Work out the finished part from the listing and answer in its coordinate system (mm). Face numbers are marked on the shaded views. Round coordinates to 2 decimals unless told otherwise and drop trailing zeros. Write each loop counter-clockwise with the first axis right and the second up, starting at its lowest first coordinate (ties: lowest second). Pieces come first, ordered by that corner, then holes.
1. Determine the mould class of the marked faces 1, 2 and 3 for opening direction X: pulls with the +X half, pulls with the -X half, needs draft (parallel to the pull), parting line crosses it, or undercut.
2. Straight lines are drawn through the part: probe 1 along Z at (x, y) = (57, -16); probe 2 along X at (y, z) = (-21, 25); probe 3 along X at (y, z) = (-22, 24). For each, find the intervals that lie inside material, in ascending order.
3. Find section C-C (y = -4). Write down the section's boundary in (x, z).
4. Find section A-A (x = 28). Write down the section's boundary in (y, z).
5. Flat-ended cylindrical pins translate along their axes: pin 1 Ø4 at (y, z) = (-20, 31.5) entering from -X; pin 2 Ø1 at (y, z) = (-24, 36.5) entering from -X; pin 3 Ø1.5 at (x, z) = (30, 15) entering from +Y. Find the tip coordinate at first contact, or state that the pin passes through.
6. Find section B-B (z = 8). Write down the section's boundary in (x, y), and give its area (3 significant figures).
7. Find section D-D (x = 54). Write down the section's boundary in (y, z), and give its area (3 significant figures).
```python
from build123d import *

# Parameters (mm, degrees)
F0_W     = 59.392195
F0_H     = 41.705828
F1_DEPTH = 3.048
F2_R     = 7.737953
F3_DEPTH = 41.656
F4_R     = 5.430673
F5_DEPTH = 50.8


with BuildPart() as f1:
    # F0 (on Top) → F1 (new body)
    with BuildSketch(Plane.XY):
        with Locations((29.696097, -20.852914)):
            Rectangle(F0_W, F0_H)
    extrude(amount=F1_DEPTH)

    # F2 (on face) → F3 (join)
    with BuildSketch(Plane.XY.offset(3.048)):
        with Locations((23.27165, -19.919522)):
            Circle(F2_R)
    extrude(amount=F3_DEPTH)

    # F4 (on face) → F5 (cut)
    with BuildSketch(Plane.XY.offset(44.704)):
        with Locations((23.27165, -19.919522)):
            Circle(F4_R)
    extrude(amount=-F5_DEPTH, mode=Mode.SUBTRACT)


solid = f1.part
```
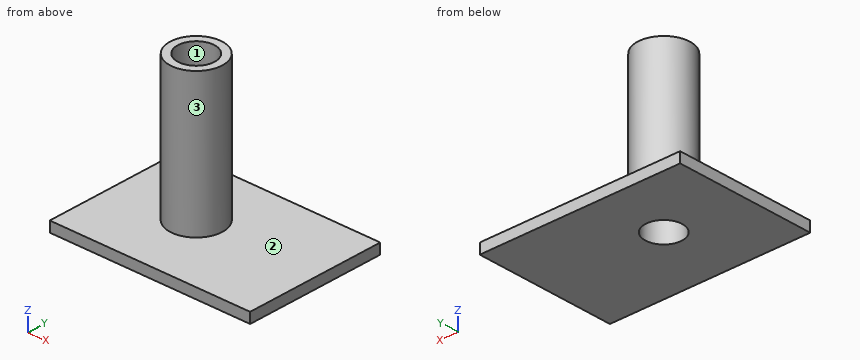
Worked answers:
1. face 1: undercut
1. face 2: needs draft
1. face 3: parting line crosses it
2. probe 1: z = 0 to 3.05
2. probe 2: x = 15.61 to 17.95, 28.59 to 30.93
2. probe 3: x = 15.82 to 18.26, 28.29 to 30.72
3. outline: (0, 0) - (59.39, 0) - (59.39, 3.05) - (0, 3.05) - close
4. outline: (-41.71, 0) - (-22.59, 0) - (-22.59, 44.7) - (-26.04, 44.7) - (-26.04, 3.05) - (-41.71, 3.05) - close; (-17.25, 0) - (0, 0) - (0, 3.05) - (-13.79, 3.05) - (-13.79, 44.7) - (-17.25, 44.7) - close
5. pin 1: stops at x = 15.53
5. pin 2: stops at x = 16.41
5. pin 3: stops at y = -15.01
6. outline: circle Ø15.48 at (23.27, -19.92); hole circle Ø10.86 at (23.27, -19.92)
6. area: 95.5 mm2
7. outline: (-41.71, 0) - (0, 0) - (0, 3.05) - (-41.71, 3.05) - close
7. area: 127 mm2
